Solid Edge part; units mm, degrees
sketch "Sketch1" plane through (0, 0, 0) normal (0, 0, 1) x (1, 0, 0)
  circle A0 centre (-62.269, 22.0507) radius 70
  circle A1 centre (-62.269, 22.0507) radius 250
extrude "Protrusion1" add sketch "Sketch1" along normal blind 50
sketch "Sketch2" plane through (-62.269, 22.0507, 50) normal (0, 0, 1) x (0, 1, 0)
  line L0 (-77.9972, 104.0021) -> (-224.2944, 299.0763)
  line L1 (-224.2944, 299.0763) -> (-306.7248, 177.0877)
  line L2 (-306.7248, 177.0877) -> (-112.5833, 65)
  arc A0 (-77.9972, 104.0021) -> (-112.5833, 65) centre (0, 0) ccw
  line L3 (112.5833, -65) -> (403.4538, -232.9342)
  line L4 (403.4538, -232.9342) -> (235.7459, -314.3458)
  line L5 (235.7459, -314.3458) -> (77.9972, -104.0021)
  arc A1 (77.9972, -104.0021) -> (112.5833, -65) centre (0, 0) ccw
  line L6 (-317.1796, 0) -> (-130, 0)
  arc A2 (-130, 0) -> (15.5465, -129.0671) centre (0, 0) ccw
  line L7 (86.2059, -715.684) -> (15.5465, -129.0671)
  line L8 (-317.1796, 0) -> (86.2059, -715.684)
  arc A3 (130, 0) -> (-15.5465, 129.0671) centre (0, 0) ccw
  line L9 (-15.5465, 129.0671) -> (-39.2378, 325.7531)
  line L10 (-39.2378, 325.7531) -> (379.3774, 186.8257)
  line L11 (379.3774, 186.8257) -> (365.0673, 0)
  line L12 (130, 0) -> (365.0673, 0)
extrude "Cutout1" cut sketch "Sketch2" against normal through all
sketch "Sketch3" plane through (-62.269, 22.0507, 50) normal (0, 0, 1) x (0, 1, 0)
  line L0 (-425.8026, 139.9754) -> (-196.3739, 78.5001)
  line L1 (-196.3739, 78.5001) -> (-209.3149, 30.2039)
  line L2 (-209.3149, 30.2039) -> (-438.7436, 91.6791)
  line L3 (-438.7436, 91.6791) -> (-425.8026, 139.9754)
  line L4 (101.4208, -185.577) -> (153.5361, -315.4253)
  line L5 (153.5361, -315.4253) -> (107.134, -334.049)
  line L6 (107.134, -334.049) -> (55.0187, -204.2007)
  line L7 (55.0187, -204.2007) -> (101.4208, -185.577)
  line L8 (209.3149, -30.2039) -> (455.6, -96.1958)
  line L9 (455.6, -96.1958) -> (442.6591, -144.492)
  line L10 (442.6591, -144.492) -> (196.3739, -78.5001)
  line L11 (196.3739, -78.5001) -> (209.3149, -30.2039)
  line L12 (-161.2539, 334.6546) -> (-101.4208, 185.577)
  line L13 (-101.4208, 185.577) -> (-55.0187, 204.2007)
  line L14 (-55.0187, 204.2007) -> (-114.8518, 353.2783)
  line L15 (-114.8518, 353.2783) -> (-161.2539, 334.6546)
  dimension "D1" = 161.2539
  dimension "D2" = 101.4208
  dimension "D3" = 438.7436
  dimension "D4" = 153.5361
  dimension "D5" = 455.6
extrude "Cutout2" cut sketch "Sketch3" against normal through all
sketch "Sketch4" plane through (-62.269, 22.0507, 50) normal (0, 0, 1) x (0.3725, -0.928, 0)
  circle A0 centre (0, 0) radius 75
extrude "Cutout3" cut sketch "Sketch4" against normal blind 40
sketch "Sketch5" plane through (-331.9141, 78.0776, 25) normal (0.3725, -0.928, 0) x (0.928, 0.3725, 0)
  circle A0 centre (-0.6266, 0) radius 5
  dimension "D1" = 0.6266
extrude "ExtrudedCutout_18" cut sketch "Sketch5" along normal through all
sketch "Sketch6" plane through (-191.9716, -180.6604, 25) normal (-0.9659, 0.2588, 0) x (-0.2588, -0.9659, 0)
  circle A0 centre (0.6266, 0) radius 5
  dimension "D1" = 0.6266
extrude "ExtrudedCutout_19" cut sketch "Sketch6" against normal through all
sketch "Sketch7" plane through (221.776, -69.8543, 25) normal (0.3725, -0.928, 0) x (0.928, 0.3725, 0)
  circle A0 centre (0.6266, 0) radius 5
  dimension "D1" = 0.6266
extrude "ExtrudedCutout_20" cut sketch "Sketch7" against normal through all
sketch "Sketch8" plane through (83.8094, 220.374, 25) normal (0.9659, -0.2588, 0) x (0.2588, 0.9659, 0)
  circle A0 centre (0.6266, 0) radius 5
  dimension "D1" = 0.6266
extrude "ExtrudedCutout_21" cut sketch "Sketch8" against normal through all
properties material "Aluminum, 6061-T6"
The model under review builds one solid part; all positions refer to its coordinate system, in mm. A direction names the side the tool comes from. Round coordinates to 2 decimals unless told otherwise and drop trailing zeros. Loops run counter-clockwise (first coordinate to the right, second up) from the corner with the lowest first, then second, coordinate; pieces in that order, holes last. Notation, with made-up numbers: M 40,-24 L 65,-24 A15 ccw 65,3 Z; hole C 47,-22 d11. An arc over 180 degrees is marked long. Answer as a JSON object with one key per item and string values.
Item 1: Clearance check with flat-ended pins moving along their axes: P1, Ø10, axis at y = 112.5, z = 42, coming from the +X side; P2, Ø3, axis at x = -232.5, z = 16, coming from the -Y side; P3, Ø3, axis at x = 118.5, z = 28.5, coming from the +Y side. State where each tip first meets the part, or that it passes through.
Check sheet entries:
{"P1": "x = 129.72", "P2": "y = -106.74", "P3": "y = 158.74"}
Item 2: We need section A-A, the plane x = -70. State how many separate pieces and enclosed holes the cut face has, and give its area (3 significant figures).
Check sheet entries:
{"separate pieces": "2", "enclosed holes": "1", "area": "11,500 mm2"}
Item 3: Tool access review of faces 5 (the face through (21.316, 237.4, 30.906)), 6 (the face through (24.26, 119.07, 25.35)), 7 (the face through (137.04, 128.983, 25.35)), 8 (the face through (-124, 56, 10)), 9 (the face through (-264.06, -106.06, 24.78)): name each direction out of +Z, -Z, +X, -X, +Y, -Y from which nothing blocks a thin tool from reaching the whole face with its end or side.
Check sheet entries:
{"face 5": "+Z, -Z, +Y", "face 6": "+Z, -Z", "face 7": "+Z, -Z, +X", "face 8": "+Z", "face 9": "none"}
Item 4: We need section B-B, the plane y = -148.5. State the section outline as (x, z) points, and give its area (3 significant figures).
Check sheet entries:
{"outline": "M -160.74,0 L -62.27,0 L -62.27,50 L -160.74,50 Z", "area": "4,920 mm2"}
Item 5: For line 1 along X through (y, z) = (133, 23.5); line 2 along X through (y, z) = (-42, 31); line 3 along Y through (x, z) = (-174.5, 29), list the stretches that pass through material, from the lowest coordinate up.
Check sheet entries:
{"line 1": "-130.02 to 5.48, 85.67 to 135.89, 146.16 to 147.05", "line 2": "-303.92 to -288.97, -262.84 to -101.29, -23.25 to 50.86", "line 3": "-201.34 to -189.1, -182.88 to -172.34, -62.12 to 87.66"}
Item 6: We need section C-C, the plane x = -237. State the section outline as (y, z) points, and give its area (3 significant figures).
Check sheet entries:
{"outline": "M -108.99,0 L 1,0 L 1,50 L -108.99,50 Z", "area": "5,500 mm2"}
Item 7: The part is to be moulded in two halves that separate along Y. For faces 1 (the face through (-119, -32, 50)), 2 (the face through (149.04, 155.65, 24.65)), 3 (the face through (172.083, 68.429, 26.502)), 4 (the face through (-257.03, -56.49, 25.35)), say which applies: +Y half, -Y half, draft (parallel to the pull), parting line (faces both ways), or undercut.
Check sheet entries:
{"face 1": "draft", "face 2": "+Y half", "face 3": "undercut", "face 4": "undercut"}
